Input: part model. Units: mm. Frame: model coordinates. Face numbers are marked on the shaded views. Give positions to 0.01 mm unless a question says otherwise; leave off trailing zeros. Loops run counter-clockwise (first coordinate to the right, second up) from the corner with the lowest first, then second, coordinate; pieces in that order, holes last. Notation, with made-up numbers: M -22.75,53.5 L 27.25,53.5 A15 cw 27.25,60.5 Z; hole C 83,86 d8. An arc over 180 degrees is marked long. Answer as a JSON object with one key per item and string values. Group by question number.
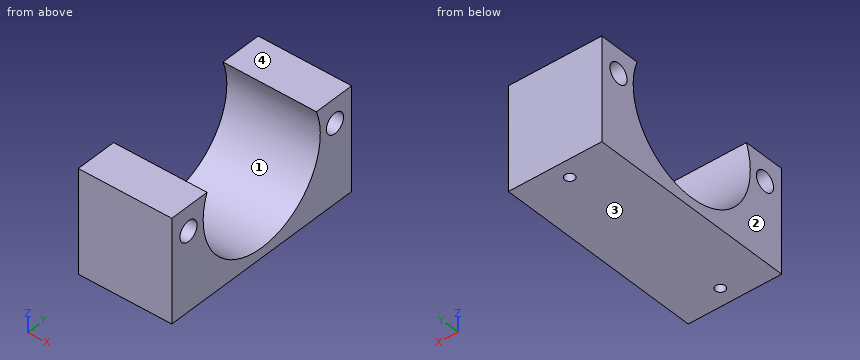
Autodesk Fusion 360 part; units mm, degrees
sketch "Sketch1" plane through (0, 0, 0) normal (1, 0, 0) x (0, 1, 0)
  line L0 (21.5, 5) -> (21.5, -16)
  line L1 (21.5, -16) -> (-21.5, -16)
  line L2 (-21.5, -16) -> (-21.5, 5)
  line L3 (-21.5, 5) -> (-13.0767, 5)
  line L4 (13.0767, 5) -> (21.5, 5)
  arc A0 (-13.0767, 5) -> (13.0767, 5) centre (0, 0) ccw
  circle A1 centre (17.5, -0.0047) radius 2.05
  circle A2 centre (-17.5, 0) radius 2.05
  dimension "d44" = 28
  dimension "d47" = 16
  dimension "d48" = 5
  dimension "d49" = 4.1
  dimension "d50" = 21.5
  dimension "d51" = 21.5
  dimension "d52" = 17.5
  dimension "d56" = 4.1
  dimension "d57" = 17.5
extrude "Extrude1" add sketch "Sketch1" along normal blind 19
sketch "Sketch2" plane through (0, 0, 0) normal (1, 0, 0) x (0, 1, 0)
  line L0 (21.5, 3.5453) -> (21.5, -0.0047)
  point P0 (15.45, -0.0047)
  point P1 (17.5, -0.0047)
  dimension "d62" = 4
sketch "Sketch3" plane through (0, 0, -16) normal (0, 0, -1) x (1, 0, 0)
  line L0 (0, 21.5) -> (0, -21.5)
  line L1 (0, -21.5) -> (19, -21.5)
  line L2 (19, -21.5) -> (19, 21.5)
  line L3 (19, 21.5) -> (0, 21.5)
  line L4 (9.5, 25) -> (9.5, -29)
  dimension "d63" = 9.5
sketch "Sketch4" plane through (0, 0, -16) normal (0, 0, -1) x (1, 0, 0)
sketch "Sketch5" plane through (0, 0, 0) normal (1, 0, 0) x (0, 1, 0)
  line L0 (-19.794, -16) -> (-15.6772, -16)
  dimension "d64" = 4.1168
  dimension "d65" = 4.1168
sketch "Sketch6" plane through (0, 0, -16) normal (0, 0, -1) x (1, 0, 0)
  circle A0 centre (9.5, 18) radius 1
  line L0 (19, 21.5) -> (0, 21.5)
  circle A1 centre (9.5, -18) radius 1
  line L1 (0, -21.5) -> (19, -21.5)
  dimension "d66" = 2
  dimension "d67" = 3.5
  dimension "d68" = 2
  dimension "d69" = 3.5
extrude "Extrude2" cut sketch "Sketch6" against normal blind 10
1. Mould query, pull axis Z, two halves, no side actions, for the marked faces 1, 2, 3 and 4. Classes: pulls with the +Z half, pulls with the -Z half, needs draft (parallel to the pull), parting line crosses it, or undercut.
2. Section A-A (z = -9.5). Output: boundary loops of the cut face in (x, y).
3. Section B-B (z = 0.5). Output: boundary loops of the cut face in (x, y), then the cut area to 3 significant figures.
4. Section D-D (x = 9.5). Output: boundary loops of the cut face in (y, z), then the cut area to 3 significant figures.
5. Section C-C (y = -16.5). Output: boundary loops of the cut face in (x, z).
6. Material intervals for L1, parallel to X at y = -18, z = -10.75; L2, parallel to Y at x = 9.5, z = -12.5; L3, parallel to Y at x = 9.5, z = -9, sorted ascending.
Geometry results:
{
 "1": {"face 1": "undercut", "face 2": "needs draft", "face 3": "pulls with the -Z half", "face 4": "pulls with the +Z half"},
 "2": {"outline": "M 0,-21.5 L 19,-21.5 L 19,-10.28 L 0,-10.28 Z; M 0,10.28 L 19,10.28 L 19,21.5 L 0,21.5 Z; hole C 9.5,-18 d2; hole C 9.5,18 d2"},
 "3": {"outline": "M 0,-21.5 L 19,-21.5 L 19,-19.49 L 0,-19.49 Z; M 0,-15.51 L 19,-15.51 L 19,-13.99 L 0,-13.99 Z; M 0,13.99 L 19,13.99 L 19,15.51 L 0,15.51 Z; M 0,19.49 L 19,19.49 L 19,21.5 L 0,21.5 Z", "area": "134 mm2"},
 "4": {"outline": "M -21.5,-16 L -19,-16 L -19,-6 L -17,-6 L -17,-16 L 17,-16 L 17,-6 L 19,-6 L 19,-16 L 21.5,-16 L 21.5,5 L 13.08,5 A14 cw long -13.08,5 L -21.5,5 Z; hole C -17.5,0 d4.1; hole C 17.5,0 d4.1", "area": "392 mm2"},
 "5": {"outline": "M 0,-16 L 19,-16 L 19,-1.79 L 0,-1.79 Z; M 0,1.79 L 19,1.79 L 19,5 L 0,5 Z"},
 "6": {"L1": "0 to 8.5, 10.5 to 19", "L2": "-21.5 to -19, -17 to -6.3, 6.3 to 17, 19 to 21.5", "L3": "-21.5 to -19, -17 to -10.72, 10.72 to 17, 19 to 21.5"}
}
